The listing builds one solid part. Answer for the finished solid, in the listing's coordinates (mm). Round coordinates to 2 decimals unless told otherwise and drop trailing zeros. Order: outer loops, then holes, each group sorted by start corner. A loop starts at its lowest first (then second) coordinate and runs counter-clockwise, first axis right, second up. Notation, with made-up numbers: M 21.25,4 L 35.25,4 A27 cw 35.25,36 Z; hole C -36,14.25 d1. An arc over 180 degrees is marked long. Put each result on its own line as item: value. Start each with the question number.
1. Consider line 1 (Z direction, x = 10, y = -169); line 2 (Z direction, x = 7, y = -137.5); line 3 (Y direction, x = 1.25, z = -221). Determine where each line is inside the solid, lowest interval first.
2. The part is cut by section B-B (z = -377). Give the vertices of the cut face in (x, y).
3. The mould has two halves that part along Z. Classify faces 1 (the face through (6, -72, -450)), 2 (the face through (6, 0, -237)), 3 (the face through (6, -115, -71)): +Z half, -Z half, draft (parallel to the pull), parting line (faces both ways), or undercut.
4. The part is cut by section A-A (z = -291.5). Give the vertices of the cut face in (x, y).
5. The part is cut by section C-C (y = -88.5). Give the vertices of the cut face in (x, z), then the cut area to 3 significant figures.
6. The part is cut by section D-D (z = -151). Give the vertices of the cut face in (x, y).
from build123d import *

# Parameters (mm, degrees)
CROQUIS1_W              = 480
CROQUIS1_H              = 310
CROQUIS1_W_2            = 28
CROQUIS1_H_2            = 12
CROQUIS1_H_3            = 11
CROQUIS1_W_3            = 30
CROQUIS1_H_4            = 30
CROQUIS1_W_4            = 59.55
CROQUIS1_H_5            = 39.8
SALIENTE_EXTRUIR1_DEPTH = 12
CROQUIS6_R              = 1.5
CORTAR_EXTRUIR2_DEPTH   = 12


with BuildPart() as part:
    # Croquis1 → Saliente-Extruir1 (new body)
    with BuildSketch(Plane(origin=(0, 0, 0), x_dir=(0, 0, -1), z_dir=(1, 0, 0))):
        with Locations((240, -155)):
            Rectangle(CROQUIS1_W, CROQUIS1_H)
        Polygon((30, -30), (450, -30), (450, -115), (369.8, -115), (369.8, -195), (450, -195), (450, -280), (30, -280), (30, -195), (110.2, -195), (110.2, -115), (30, -115), align=None, mode=Mode.SUBTRACT)
        with Locations((282.300325034, -295)):
            Rectangle(CROQUIS1_W_2, CROQUIS1_H_2, mode=Mode.SUBTRACT)
        with Locations((234.300325034, -294.5)):
            Rectangle(CROQUIS1_W_2, CROQUIS1_H_3, mode=Mode.SUBTRACT)
        with Locations((186.300325034, -295)):
            Rectangle(CROQUIS1_W_2, CROQUIS1_H_2, mode=Mode.SUBTRACT)
        with Locations((186.300325034, -15)):
            Rectangle(CROQUIS1_W_2, CROQUIS1_H_2, mode=Mode.SUBTRACT)
        with Locations((282.300325034, -15)):
            Rectangle(CROQUIS1_W_2, CROQUIS1_H_2, mode=Mode.SUBTRACT)
        with Locations((234.300325034, -15.5)):
            Rectangle(CROQUIS1_W_2, CROQUIS1_H_3, mode=Mode.SUBTRACT)
        with Locations((45, -155)):
            Rectangle(CROQUIS1_W_3, CROQUIS1_H_4, mode=Mode.SUBTRACT)
        with Locations((420.225, -155)):
            Rectangle(CROQUIS1_W_4, CROQUIS1_H_5, mode=Mode.SUBTRACT)
    extrude(amount=SALIENTE_EXTRUIR1_DEPTH)

    # Croquis6 → Cortar-Extruir2 (cut)
    with BuildSketch(Plane(origin=(12, 0, 0), x_dir=(0, 0, -1), z_dir=(1, 0, 0))):
        with Locations((173.24106245, -19.831662243)):
            Circle(CROQUIS6_R)
        with Locations((199.239664862, -19.939339828)):
            Circle(CROQUIS6_R)
    extrude(amount=-CORTAR_EXTRUIR2_DEPTH, mode=Mode.SUBTRACT)


solid = part.part
Resolved:
1. line 1: -480 to -450, -390.45 to -369.8, -110.2 to -60, -30 to 0
1. line 2: -480 to -450, -390.45 to -369.8, -110.2 to 0
1. line 3: -310 to -300, -289 to -280, -30 to -21, -10 to 0
2. outline: M 0,-310 L 12,-310 L 12,-280 L 0,-280 Z; M 0,-195 L 12,-195 L 12,-115 L 0,-115 Z; M 0,-30 L 12,-30 L 12,0 L 0,0 Z
3. face 1: undercut
3. face 2: draft
3. face 3: undercut
4. outline: M 0,-310 L 12,-310 L 12,-301 L 0,-301 Z; M 0,-289 L 12,-289 L 12,-280 L 0,-280 Z; M 0,-30 L 12,-30 L 12,-21 L 0,-21 Z; M 0,-9 L 12,-9 L 12,0 L 0,0 Z
5. outline: M 0,-480 L 12,-480 L 12,-450 L 0,-450 Z; M 0,-30 L 12,-30 L 12,0 L 0,0 Z
5. area: 720 mm2
6. outline: M 0,-310 L 12,-310 L 12,-280 L 0,-280 Z; M 0,-30 L 12,-30 L 12,0 L 0,0 Z
